Source: CAD feature listing. Evaluate the final solid. Frame: model axes, mm. Face numbers are marked on the shaded views. A direction names the side the tool comes from. Coordinates: 2 decimals unless noted, no trailing zeros. Loops run counter-clockwise (first coordinate to the right, second up) from the corner with the lowest first, then second, coordinate; pieces in that order, holes last. Notation, with made-up numbers: (82.5, 43.5) - (130.5, 43.5) arc R14 ccw to (130.5, 63.5) - close; hole circle Ø4 at (31, 82.5). An arc over 180 degrees is marked (long way). Use one line per item in the form item = value. Start each with the question number.
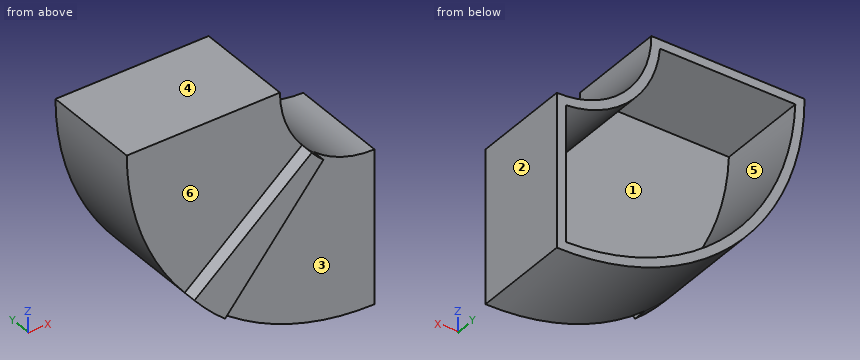
from build123d import *

# Parameters (mm, degrees)
ESTRUSIONE_ESTRUSIONE1_DEPTH = 3
ESTRUSIONE_SOTTILE1_DEPTH    = 44
ESTRUSIONE_ESTRUSIONE2_START = 6
ESTRUSIONE_ESTRUSIONE2_DEPTH = 6


with BuildPart() as part:
    # Schizzo1 → Estrusione-Estrusione1 (new body)
    with BuildSketch(Plane(origin=(0, 0, 0), x_dir=(1, 0, 0), z_dir=(0, 1, 0))):
        with BuildLine():
            Line((-110, 0), (-42, 0))
            ThreePointArc((-42, 0), (-29.69848481, 29.69848481), (0, 42))
            Line((0, 42), (0, 110))
            ThreePointArc((0, 110), (-77.781745931, 77.781745931), (-110, 0))
        make_face()
    extrude(amount=ESTRUSIONE_ESTRUSIONE1_DEPTH)

    # Schizzo1<2> → Estrusione-Sottile1 (add)
    with BuildSketch(Plane(origin=(0, 0, 0), x_dir=(1, 0, 0), z_dir=(0, 1, 0))):
        with BuildLine():
            Line((0, 42), (0, 110))
            ThreePointArc((0, 110), (-77.781745931, 77.781745931), (-110, 0))
            Line((-110, 0), (-42, 0))
            ThreePointArc((-42, 0), (-29.69848481, 29.69848481), (0, 42))
        make_face()
        with BuildLine():
            Line((-4, 45.82575695), (-4, 105.924501415))
            ThreePointArc((-4, 105.924501415), (-74.953318806, 74.953318806), (-105.924501415, 4))
            Line((-105.924501415, 4), (-45.82575695, 4))
            ThreePointArc((-45.82575695, 4), (-32.526911935, 32.526911935), (-4, 45.82575695))
        make_face(mode=Mode.SUBTRACT)
    extrude(amount=ESTRUSIONE_SOTTILE1_DEPTH)

    # Schizzo2 → Estrusione-Estrusione2 (add)
    with BuildSketch(Plane.XZ.offset(ESTRUSIONE_ESTRUSIONE2_START)):
        with BuildLine():
            Line((-84.264888743, -70.706637066), (-32.173866611, -26.997079607))
            ThreePointArc((-32.173866611, -26.997079607), (-29.69848481, -29.69848481), (-26.997079607, -32.173866611))
            Line((-26.997079607, -32.173866611), (-70.706637066, -84.264888743))
            ThreePointArc((-70.706637066, -84.264888743), (-77.781745931, -77.781745931), (-84.264888743, -70.706637066))
        make_face()
    extrude(amount=-ESTRUSIONE_ESTRUSIONE2_DEPTH)


solid = part.part
(1) Cut plane B-B, the plane z = -62. Output: boundary loops of the cut face in (x, y).
(2) Material intervals for line 1 (Y direction, x = -71, z = -11.5); line 2 (Z direction, x = -71.5, y = 28.5); line 3 (Z direction, x = -15, y = 11.5), sorted ascending.
(3) Mould query, pull axis Z, two halves, no side actions, for the marked faces 4, 5 and 6. Classes: +Z half, -Z half, draft (parallel to the pull), parting line (faces both ways), or undercut.
(4) Contact query for flat-ended pins moving along their axis: pin 1 (1.5 mm diameter, centred on y = 15.5, z = -84.5, fed in from -X); pin 2 (10 mm diameter, centred on y = 28, z = -33.5, fed in from +X); pin 3 (3 mm diameter, centred on x = -37, z = -68.5, fed in from +Y). Output: stop coordinate, or through.
(5) Access query for the marked faces 1, 2 and 3. Directions: +Z, -Z, +X, -X, +Y, -Y. A direction counts if a zero-diameter tool reaches every point of the face in a straight line with its end or side. Return the directions, or none.
(6) Cut plane D-D, the plane y = -2. Output: boundary loops of the cut face in (x, z).
(7) Cut plane C-C, the plane x = -86.5. Output: boundary loops of the cut face in (y, z).
(8) Cut plane A-A, the plane y = 32. Output: boundary loops of the cut face in (x, z), plus the area to 3 significant figures.
Recorded:
q1.outline = (-90.86, 0) - (-73.89, 0) - (-73.89, -6) - (-52.02, -6) - (-52.02, 0) - (0, 0) - (0, 44) - (-4, 44) - (-4, 3) - (-85.98, 3) - (-85.98, 44) - (-90.86, 44) - close
q2.line_1 = 0 to 3
q2.line_2 = -83.59 to -78.25, -4 to 0
q2.line_3 = -108.97 to -104.93, -43.49 to -39.23
q3.face_4 = +Z half
q3.face_5 = undercut
q3.face_6 = draft
q4.pin_1 = -71.32
q4.pin_2 = -16.79
q4.pin_3 = 3
q5.face_1 = +Y
q5.face_2 = +Z, -Z, +X, +Y, -Y
q5.face_3 = -Z, +X, -Y
q6.outline = (-84.26, -70.71) arc R110 ccw to (-70.71, -84.26) - (-27, -32.17) arc R42 cw to (-32.17, -27) - close
q7.outline = (0, -67.95) - (44, -67.95) - (44, -61.27) - (3, -61.27) - (3, -4) - (44, -4) - (44, 0) - (0, 0) - close
q8.outline = (-110, 0) arc R110 ccw to (0, -110) - (0, -42) arc R42 cw to (-42, 0) - close; hole (-105.92, -4) arc R106 ccw to (-4, -105.92) - (-4, -45.83) arc R46 cw to (-45.83, -4) - close
q8.area = 1,440 mm²
